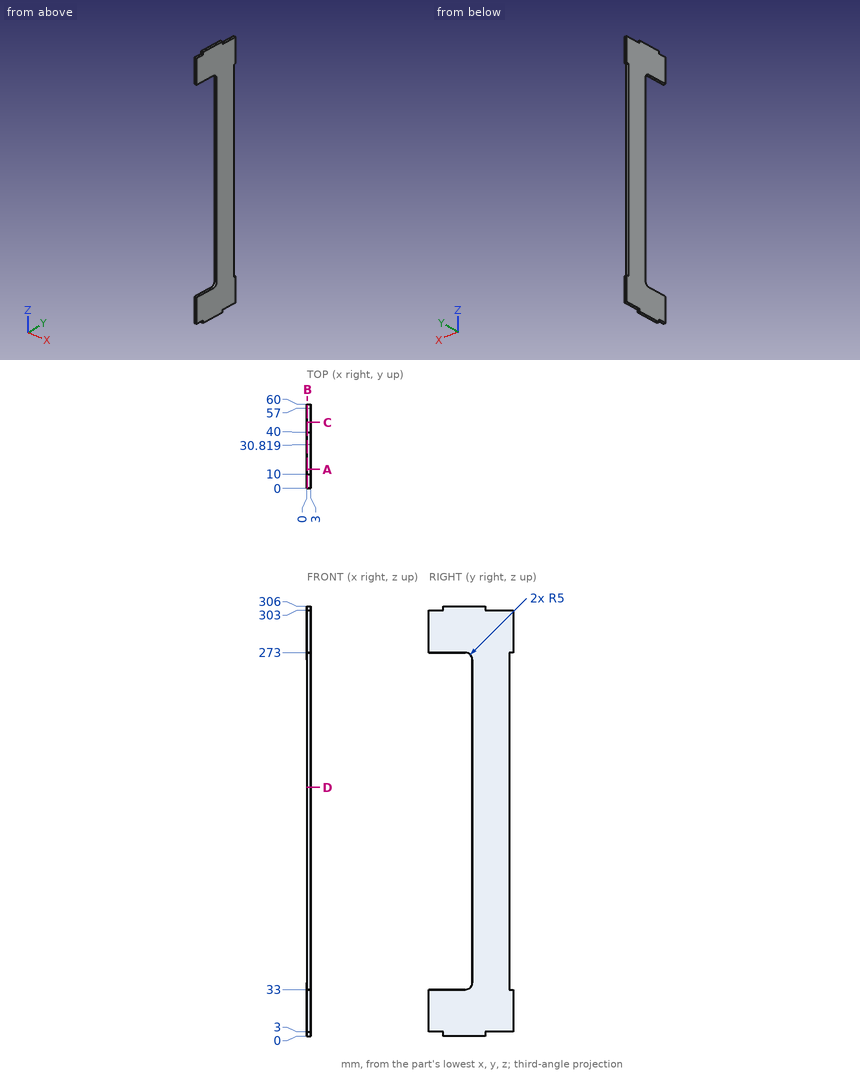
Could you check a few things on this drawing? It's one solid part, dimensions in mm from its lowest x, y, z. Coordinates: 2 decimals unless noted, no trailing zeros. Write each loop counter-clockwise with the first axis right and the second up, starting at its lowest first coordinate (ties: lowest second). Pieces come first, ordered by that corner, then holes. Notation, with made-up numbers: (-7.5, 42) - (9.5, 42) arc R36 ccw to (9.5, 80) - close; hole circle Ø1 at (81, -25.5). An arc over 180 degrees is marked (long way). Write item = value, one per line.
1) Suppose I cut it at B-B on x = 0.45. Please give me the cut outline in (y, z), plus the area to 3 significant figures.
Result set:
outline = (0, 3) - (10, 3) - (10, 0) - (40, 0) - (40, 3) - (60, 3) - (60, 33) - (57, 33) - (57, 273) - (60, 273) - (60, 303) - (40, 303) - (40, 306) - (10, 306) - (10, 303) - (0, 303) - (0, 273) - (25.82, 273) arc R5 cw to (30.82, 268) - (30.82, 38) arc R5 cw to (25.82, 33) - (0, 33) - close
area = 10,100 mm2
2) Suppose I cut it at A-A on y = 13.5. Please give me the cut outline in (x, z).
Result set:
outline = (0, 0) - (3, 0) - (3, 33) - (0, 33) - close; (0, 273) - (3, 273) - (3, 306) - (0, 306) - close
3) Will these pins go through, and if not, where does the flat tip stop? pin 1 Ø0.9 at (x, z) = (1.5, 1) entering from -Y; pin 2 Ø0.9 at (x, y) = (1.5, 58.5) entering from +Z; pin 3 Ø0.9 at (x, y) = (2, 3) entering from -Z.
Result set:
pin_1 = 10
pin_2 = 303
pin_3 = 3
4) Suppose I cut it at D-D on z = 177. Please give me the cut outline in (x, y), plus the area to 3 significant figures.
Result set:
outline = (0, 30.82) - (3, 30.82) - (3, 57) - (0, 57) - close
area = 78.5 mm2
5) Please list where these lines run through material, in increasing order: line 1 (Z direction, x = 0.6, y = 25.5); line 2 (Z direction, x = 2.2, y = 46); line 3 (Z direction, x = 1.1, y = 8.5). Write a range as [from, to].
Result set:
line_1 = [0, 33], [273, 306]
line_2 = [3, 303]
line_3 = [3, 33], [273, 303]
6) Suppose I cut it at C-C on y = 47. Please give me the cut outline in (x, z), plus the area to 3 significant figures.
Result set:
outline = (0, 3) - (3, 3) - (3, 303) - (0, 303) - close
area = 900 mm2
